Check sheet for the modelled part. Datum: model origin and axes. Units: mm. A direction names the side the tool comes from. Round coordinates to 2 decimals unless told otherwise and drop trailing zeros. Order: outer loops, then holes, each group sorted by start corner. A loop starts at its lowest first (then second) coordinate and runs counter-clockwise, first axis right, second up.
(1) Sectioned sample at B-B, the plane z = 12.7. Enter the section's corners in (x, y) (1 decimal).
(2) Thickness scan on probe 1 along Z at (x, y) = (3.75, 4.75); probe 2 along Z at (x, y) = (12.7, -2.25) (3 decimals); probe 3 along X at (y, z) = (-2.4, 12.7) (1 decimal). Record the ranges inside material, lowest first.
(3) Tool access check on faces 1 (the flat face through (13, 6, 1.588)), 2 (the cylindrical face through (0.084, -2.392, 6.33)). Record the directions out of +Z, -Z, +X, -X, +Y, -Y that give a thin tool (end or side, any length) a straight path to the whole face; none if there is none.
(4) Sectioned sample at C-C, the plane y = 5.25. Enter the section's corners in (x, z).
(5) Mould release check, pull along X, two halves, no side actions. Record for faces 3 (the flat face through (13, 12.7, 1)), 4 (the flat face through (0, 2, 1)), 5 (the cylindrical face through (16.563, 6.241, 0.783)): released by +X, released by -X, zero draft, split by the parting line, or undercut.
(6) Depth check by flat-ended pin: pin 1 (4 mm diameter, centred on y = -1, z = 15, fed in from -X); pin 2 (6 mm diameter, centred on x = 4, z = 13, fed in from +Y); pin 3 (5 mm diameter, centred on x = 12.7, z = 12.7, fed in from +Y); pin 4 (6.5 mm diameter, centred on x = 12, y = 5, fed in from +Z). Enter the tip coordinate at first touch or a pass-through.
Autodesk Inventor part; units mm, degrees
ref_plane "YZ Plane" through (0, 0, 0) normal (1, 0, 0) x (0, 1, 0)
ref_plane "XZ Plane" through (0, 0, 0) normal (0, 1, 0) x (-1, 0, 0)
ref_plane "XY Plane" through (0, 0, 0) normal (0, 0, 1) x (1, 0, 0)
sketch "Sketch1" plane through (0, 0, 0) normal (0, 0, 1) x (1, 0, 0)
  line L0 (0, 0) -> (25.4, 0)
  line L1 (25.4, 0) -> (25.4, 12.7)
  line L2 (25.4, 12.7) -> (0, 12.7)
  line L3 (0, 12.7) -> (0, 0)
  circle A0 centre (6.35, 6.35) radius 2.4892
  circle A1 centre (19.05, 6.35) radius 2.4892
  line L4 (12.7, 12.7) -> (12.7, 0) construction
  dimension "d0" = 25.4
  dimension "d1" = 12.7
  dimension "d2" = 4.9784
  dimension "d3" = 4.9784
  dimension "d4" = 6.35
  dimension "d5" = 6.35
  dimension "d6" = 6.35
  dimension "d7" = 6.35
extrude "Plate1" add sketch "Sketch1" along normal blind 1.5875
sketch "Sketch2" plane through (25.4, -1.5875, 3.175) normal (0, -1, 0) x (1, 0, 0)
  line L0 (-25.4, 0) -> (0, 0)
  line L1 (0, 0) -> (0, 15.875)
  line L2 (0, 15.875) -> (-25.4, 15.875)
  line L3 (-25.4, 15.875) -> (-25.4, 0)
edge flange "Flange1" height 19.05 angle 90 thickness 1.5875 bend radius 1.5875 thickness toward (0, -1, 0) relief tear relief width 1.5875 relief depth 0.7937 edges at (12.7, 0, 1.5875) wall of the first edge with corners at (0, -1.5875, 3.175) (25.4, -1.5875, 3.175) (25.4, -1.5875, 19.05) (0, -1.5875, 19.05)
bend "Bend1"
corner "Corner1"
sketch "Sketch3" plane through (0, -1.5875, 19.05) normal (0, 1, 0) x (1, 0, 0)
  line L0 (25.4, 15.875) -> (0, 15.875)
  line L1 (0, 0) -> (0, 15.875)
  line L2 (0, 0) -> (25.4, 0)
  line L3 (25.4, 0) -> (25.4, 15.875)
  line L4 (0, 12.7) -> (9.525, 0)
  line L5 (12.7, 0) -> (12.7, 15.875) construction
  line L6 (25.4, 12.7) -> (15.875, 0)
  circle A0 centre (12.7, 6.35) radius 3.175
  line L7 (9.525, 0) -> (15.875, 0)
  line L8 (25.4, 12.7) -> (25.4, 15.875)
  point P0 (0, 19.05)
  dimension "d19" = 3.175
  dimension "d20" = 3.175
  dimension "d21" = 6.35
  dimension "d22" = 6.35
extrude "Extrusion1" cut sketch "Sketch3" against normal blind 25.4 contours L3 L2 L6 | L4 L2 L1 | A0
fillet "Fillet1" radius 1.5875 6 edges at (9.525, -2.3812, 19.05) (0, -2.3813, 6.35) (25.4, -2.3813, 6.35) (15.875, -2.3812, 19.05) (25.4, 12.7, 0.7937) (0, 12.7, 0.7937)
equation "\"d5\" = d4"
equation "\"d7\" = d6"
equation "\"d9\" = BendReliefWidth"
equation "\"d10\" = BendReliefDepth"
equation "\"d11\" = MinimumRemnant"
equation "\"d12\" = BendRadius"
equation "\"d15\" = BendRadius"
equation "\"d16\" = CornerReliefSize"
equation "\"d17\" = GapSize"
equation "\"d18\" = JacobiRadiusSize"
equation "\"BendRadius\" = Thickness"
equation "\"BendReliefWidth\" = Thickness"
equation "\"BendReliefDepth\" = 0.5 * Thickness"
equation "\"CornerReliefSize\" = 4 * Thickness"
equation "\"MinimumRemnant\" = 2 * Thickness"
equation "\"TransitionRadius\" = BendRadius"
equation "\"JacobiRadiusSize\" = BendRadius"
equation "\"GapSize\" = Thickness"
equation "\"d8\" = BendRadius"
properties part number "Flange for Torsion Spring" material "Aluminum"
Derived:
1. outline: (4.8, -3.2) - (9.5, -3.2) - (9.5, -1.6) - (4.8, -1.6) - close; (15.9, -3.2) - (20.6, -3.2) - (20.6, -1.6) - (15.9, -1.6) - close
2. probe 1: z = 0 to 1.59
2. probe 2: z = 0.935 to 9.525, 15.875 to 19.05
2. probe 3: x = 4.8 to 9.5, 15.9 to 20.6
3. face 1: +Z, +X, -X, +Y
3. face 2: +Z, -X, +Y, -Y
4. outline: (0, 0) - (4.12, 0) - (4.12, 1.59) - (0, 1.59) - close; (8.58, 0) - (16.82, 0) - (16.82, 1.59) - (8.58, 1.59) - close; (21.28, 0) - (25.4, 0) - (25.4, 1.59) - (21.28, 1.59) - close
5. face 3: zero draft
5. face 4: released by -X
5. face 5: undercut
6. pin 1: stops at x = 5.05
6. pin 2: stops at y = -1.59
6. pin 3: passes through
6. pin 4: stops at z = 1.59
